from build123d import *

# Parameters (mm, degrees)
SKETCH_1_W      = 23.2
SKETCH_1_H      = 67
EXTRUDE_1_DEPTH = 30.5
FILLET_2_R      = 2
SKETCH_2_R      = 1
SKETCH_2_R_2    = 0.5
EXTRUDE_2_DEPTH = 2


with BuildPart() as part:
    # Эскиз1 → Бобышка-Вытянуть1 (new body)
    with BuildSketch(Plane(origin=(0, 0, 0), x_dir=(1, 0, 0), z_dir=(0, 1, 0))):
        Rectangle(SKETCH_1_W, SKETCH_1_H)
    extrude(amount=EXTRUDE_1_DEPTH)

    # Скругление2
    fillet_2_edges = [part.edges().sort_by_distance(p)[0] for p in [
        (-11.6, 30.5, 0),
        (0, 30.5, 33.5),
        (11.6, 30.5, 0),
        (0, 0, 33.5),
        (-11.6, 0, 0),
        (0, 0, -33.5),
        (11.6, 0, 0),
        (0, 30.5, -33.5),
        (11.6, 15.25, 33.5),
        (-11.6, 15.25, 33.5),
        (-11.6, 15.25, -33.5),
        (11.6, 15.25, -33.5),
    ]]
    fillet(fillet_2_edges, radius=FILLET_2_R)

    # Эскиз2 → Бобышка-Вытянуть2 (add)
    with BuildSketch(Plane(origin=(0, 0, -33.5), x_dir=(-1, 0, 0), z_dir=(0, 0, -1))):
        with Locations((-1.6, 28.5)):
            Circle(SKETCH_2_R)
        with Locations((1.6, 28.5)):
            Circle(SKETCH_2_R)
        with Locations(Location((-0.6, 4.698268405, 0), (0, 0, 180))):
            Circle(SKETCH_2_R_2)
        with Locations(Location((-2.1, 4.698268405, 0), (0, 0, 180))):
            Circle(SKETCH_2_R_2)
        with Locations(Location((0.6, 4.698268405, 0), (0, 0, 180))):
            Circle(SKETCH_2_R_2)
        with Locations(Location((2.1, 4.698268405, 0), (0, 0, 180))):
            Circle(SKETCH_2_R_2)
    extrude(amount=EXTRUDE_2_DEPTH)


solid = part.part
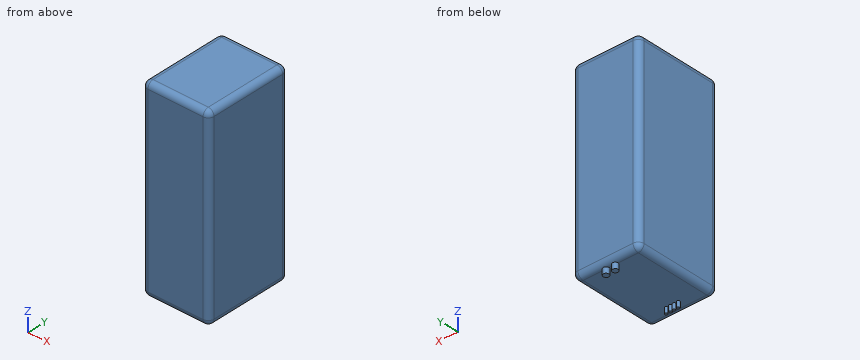
Read the model definition and answer for the solid it produces. Units are mm, in the model's axes. Coordinates: 2 decimals unless noted, no trailing zeros. Loops run counter-clockwise (first coordinate to the right, second up) from the corner with the lowest first, then second, coordinate; pieces in that order, holes last.
Q1. The part is cut by section A-A on x = -6.25. Write down the section's boundary in (y, z), and give its area (3 significant figures).
Q2. Each of these flat-tipped pins is pushed along its axis until it touches: pin 1 Ø0.5 at (x, y) = (-1.5, 29) entering from +Z; pin 2 Ø1 at (x, y) = (3, 10.5) entering from -Z. Where does it stop, or does it pass through?
Q3. The part is cut by section B-B on y = 3. Write down the section's boundary in (x, z).
Q4. Consider probe 1 along Z at (x, y) = (8, 14); probe 2 along X at (y, z) = (1.5, -27); probe 3 along Z at (x, y) = (-10.5, 25). Determine where each line is inside the solid, lowest interval first.
Results below:
1. outline: (0, -31.5) arc R2 ccw to (2, -33.5) - (28.5, -33.5) arc R2 ccw to (30.5, -31.5) - (30.5, 31.5) arc R2 ccw to (28.5, 33.5) - (2, 33.5) arc R2 ccw to (0, 31.5) - close
1. area: 2,040 mm2
2. pin 1: stops at z = 33.48
2. pin 2: stops at z = -33.5
3. outline: (-11.6, -31.5) arc R2 ccw to (-9.6, -33.5) - (9.6, -33.5) arc R2 ccw to (11.6, -31.5) - (11.6, 31.5) arc R2 ccw to (9.6, 33.5) - (-9.6, 33.5) arc R2 ccw to (-11.6, 31.5) - close
4. probe 1: z = -33.5 to 33.5
4. probe 2: x = -11.54 to 11.54
4. probe 3: z = -33.29 to 33.29
